Design review of the part built by this model. Coordinates are the model's own, in mm. A direction names the side the tool comes from. Round coordinates to 2 decimals unless told otherwise and drop trailing zeros. Loops run counter-clockwise (first coordinate to the right, second up) from the corner with the lowest first, then second, coordinate; pieces in that order, holes last. Notation, with made-up numbers: (33.5, 5.25) -> (40.5, 5.25) arc R7 ccw to (40.5, 12.25) -> close; hole circle Ø10 at (36, 2.5). An arc over 180 degrees is marked (long way). Use a Markdown table: item, result. Add a question column.
from build123d import *

# Parameters (mm, degrees)
SKETCH1_W            = 6.185857864
SKETCH1_H            = 7.5
BOSS_EXTRUDE1_DEPTH  = 4
FILLET1_R            = 2
M3_CLEARANCE_HOLE1_D = 3.2
SKETCH4_W            = 2
SKETCH4_H            = 0.481048
SKETCH4_H_2          = 1
CUT_EXTRUDE1_DEPTH   = 10
FILLET2_R            = 10
FILLET3_R            = 1
FILLET4_R            = 1


with BuildPart() as part:
    # Sketch1 → Boss-Extrude1 (new body)
    with BuildSketch(Plane.XY):
        Polygon((-4.235857864, -11.50026715), (-4.235857864, 0.5), (-19.56054874, 0.5), (-19.56054874, 9.2), (16.83945126, 9.2), (16.83945126, 0.5), (13.95, 0.5), (13.95, -7), (27.186678327, -7), (28.517391444, -8.547881241), (28.517391444, -11.5), align=None)
        with Locations((4.857071068, -3.25)):
            Rectangle(SKETCH1_W, SKETCH1_H, mode=Mode.SUBTRACT)
    extrude(amount=BOSS_EXTRUDE1_DEPTH)

    # Fillet1
    fillet1_edges = [part.edges().sort_by_distance(p)[0] for p in [
        (1.764142136, -7, 2),
        (7.95, -7, 2),
        (-4.235857864, -11.50026715, 2),
        (13.95, -7, 2),
        (28.517391444, -11.5, 2),
    ]]
    fillet(fillet1_edges, radius=FILLET1_R)

    # M3 Clearance Hole1 (through all)
    with Locations(Plane.XY.offset(4)):
        with Locations((10.95, -2.5), (-1.235857864, -2.5), (11.502527164, 5.109476), (-15.36054874, 5.109476)):
            Hole(M3_CLEARANCE_HOLE1_D / 2)

    # Sketch4 → Cut-Extrude1 (cut)
    with BuildSketch(Plane.XY.offset(4)):
        with Locations((8.502527164, 8.959476)):
            Rectangle(SKETCH4_W, SKETCH4_H)
        with Locations((-12.36054874, 8.959476)):
            Rectangle(SKETCH4_W, SKETCH4_H)
        with Locations((-12.36054874, 1)):
            Rectangle(SKETCH4_W, SKETCH4_H_2)
        Polygon((7.502527164, 0.5), (7.502527164, 1.5), (9.502527164, 1.5), (9.502527164, 0.5), (9.502527164, 0), (7.502527164, 0), align=None)
    extrude(amount=-CUT_EXTRUDE1_DEPTH, mode=Mode.SUBTRACT)

    # Fillet2
    # the kernel refuses this fillet: 10 mm, written as the material it takes off along each edge
    with BuildSketch(Plane(origin=(7.502527164, 0.5, -10.897247359), x_dir=(-1, 0, 0), z_dir=(0, 0, 1))) as fillet2_piece_1:
        with BuildLine():
            CenterArc((4.358898944, -10), FILLET2_R, 90, 25.841932763)
            Line((0, -1), (0, 0))
            Line((0, 0), (4.358898944, 0))
        make_face()
    extrude(amount=25.794494718, mode=Mode.SUBTRACT)
    with BuildSketch(Plane(origin=(7.95, 0, 16.650074726), x_dir=(1.0, -2.8096218791575343e-12, 0), z_dir=(0, 0, -1))) as fillet2_piece_2:
        with BuildLine():
            CenterArc((9.994593415, 5.36017886), FILLET2_R, 181.719985699, 30.692982598)
            Line((-0.000901098, 5.06002981), (-1.000450549, 5.030014905))
            ThreePointArc((-1.000450549, 5.030014905), (-1, 5), (-1, 0))
            Line((-1, 0), (0, -1))
            ThreePointArc((0, -1), (0.776263582, -1), (0.708320539, -0.536017886))
            Line((0.708320539, -0.536017886), (1.552527164, 0))
        make_face()
    extrude(amount=29.300149451, mode=Mode.SUBTRACT)

    # Fillet3
    # the kernel refuses this fillet: 1 mm, written as the material it adds along each edge
    with BuildSketch(Plane(origin=(9.502527164, 0, 4), x_dir=(0, 1, 0), z_dir=(0, 0, -1))) as fillet3_piece_1:
        with BuildLine():
            CenterArc((0.283169872, -1), FILLET3_R, 90, 30.865981789)
            ThreePointArc((-0.229861831, -0.141630341), (-0.114452906, -0.071590966), (0, 0))
            Line((0, 0), (0.283169872, 0))
        make_face()
    extrude(amount=4)
    with BuildSketch(Plane(origin=(9.502527164, 1.5, 4), x_dir=(-1, 0, 0), z_dir=(0, 0, -1))) as fillet3_piece_2:
        with BuildLine():
            CenterArc((FILLET3_R, -FILLET3_R), FILLET3_R, 90, 90)
            Line((0, -FILLET3_R), (0, 0))
            Line((0, 0), (FILLET3_R, 0))
        make_face()
    extrude(amount=4)
    with BuildSketch(Plane(origin=(7.502527164, 1.5, 4), x_dir=(-0.9045968857212806, -0.42626807802527333, 0), z_dir=(0, 0, -1))) as fillet3_piece_3:
        with BuildLine():
            CenterArc((0.223930785, -0.999943145), FILLET3_R, 90.610977717, 24.619977329)
            Line((-0.202337293, -0.095346259), (0, 0))
            ThreePointArc((0, 0), (0.106633707, -0.000568554), (0.213267415, 0))
        make_face()
    extrude(amount=4)
    with BuildSketch(Plane(origin=(-13.36054874, 8.718952, 4), x_dir=(0, 1, 0), z_dir=(0, 0, -1))) as fillet3_piece_4:
        with BuildLine():
            CenterArc((1, 0.854803382), FILLET3_R, 180, 58.738020049)
            Line((0, 0.854803382), (0, 0))
            Line((0, 0), (0.481048, 0))
        make_face()
    extrude(amount=4)
    with BuildSketch(Plane(origin=(-11.36054874, 8.718952, 4), x_dir=(-1, 0, 0), z_dir=(0, 0, -1))) as fillet3_piece_5:
        with BuildLine():
            CenterArc((0.854803382, 1), FILLET3_R, 211.261979951, 58.738020049)
            Line((0, 0.481048), (0, 0))
            Line((0, 0), (0.854803382, 0))
        make_face()
    extrude(amount=4)
    with BuildSketch(Plane(origin=(9.502527164, 8.718952, 4), x_dir=(0, 1, 0), z_dir=(0, 0, -1))) as fillet3_piece_6:
        with BuildLine():
            CenterArc((1, -0.854803382), FILLET3_R, 121.261979951, 58.738020049)
            Line((0, -0.854803382), (0, 0))
            Line((0, 0), (0.481048, 0))
        make_face()
    extrude(amount=4)
    with BuildSketch(Plane(origin=(7.502527164, 8.718952, 4), x_dir=(1, 0, 0), z_dir=(0, 0, -1))) as fillet3_piece_7:
        with BuildLine():
            CenterArc((0.854803382, -1), FILLET3_R, 90, 58.738020049)
            Line((0, -0.481048), (0, 0))
            Line((0, 0), (0.854803382, 0))
        make_face()
    extrude(amount=4)
    with BuildSketch(Plane(origin=(-13.36054874, 1.5, 4), x_dir=(1, 0, 0), z_dir=(0, 0, -1)), Plane(origin=(-11.36054874, 1.5, 4), x_dir=(0, -1, 0), z_dir=(0, 0, -1))) as fillet3_piece_8:
        with BuildLine():
            CenterArc((FILLET3_R, FILLET3_R), FILLET3_R, 180, 90)
            Line((0, FILLET3_R), (0, 0))
            Line((0, 0), (FILLET3_R, 0))
        make_face()
    extrude(amount=4)
    # the kernel refuses this fillet: 1 mm, written as the material it takes off along each edge
    with BuildSketch(Plane(origin=(28.517391444, -8.547881241, -0.926902713), x_dir=(0, -1, 0), z_dir=(0, 0, 1))) as fillet3_2_piece_1:
        with BuildLine():
            CenterArc((FILLET3_R * 0.370761085346, -FILLET3_R), FILLET3_R, 90, 40.685640486)
            Line((-FILLET3_R * 0.28114729377, -FILLET3_R * 0.241702258187), (0, 0))
            Line((0, 0), (FILLET3_R * 0.370761085346, 0))
        make_face()
    extrude(amount=5.853805427, mode=Mode.SUBTRACT)
    with BuildSketch(Plane(origin=(27.186678327, -7, -1.147608656), x_dir=(0.6519083791154829, -0.7582977418132165, 0), z_dir=(0, 0, 1))) as fillet3_2_piece_2:
        with BuildLine():
            CenterArc((FILLET3_R * 0.459043462337, -FILLET3_R), FILLET3_R, 90, 49.314359514)
            Line((-FILLET3_R * 0.299254279476, -FILLET3_R * 0.348091620885), (0, 0))
            Line((0, 0), (FILLET3_R * 0.459043462337, 0))
        make_face()
    extrude(amount=6.295217312, mode=Mode.SUBTRACT)
    with BuildSketch(Plane(origin=(-19.56054874, 0.5, -2.5), x_dir=(0, 1, 0), z_dir=(0, 0, 1)), Plane(origin=(-19.56054874, 9.2, -2.5), x_dir=(1, 0, 0), z_dir=(0, 0, 1)), Plane(origin=(16.83945126, 9.2, -2.5), x_dir=(0, -1, 0), z_dir=(0, 0, 1)), Plane(origin=(16.83945126, 0.5, -2.5), x_dir=(-1, 0, 0), z_dir=(0, 0, 1))) as fillet3_2_piece_3:
        with BuildLine():
            CenterArc((FILLET3_R, -FILLET3_R), FILLET3_R, 90, 90)
            Line((0, -FILLET3_R), (0, 0))
            Line((0, 0), (FILLET3_R, 0))
        make_face()
    extrude(amount=9, mode=Mode.SUBTRACT)

    # Fillet4
    fillet4_edges = [part.edges().sort_by_distance(p)[0] for p in [
        (9.502527164, 9.2, 2),
        (7.502527164, 9.2, 2),
        (-11.36054874, 9.2, 2),
        (-13.36054874, 9.2, 2),
        (-13.36054874, 0.5, 2),
        (-11.36054874, 0.5, 2),
    ]]
    fillet(fillet4_edges, radius=FILLET4_R)


solid = part.part
1. Insertion check: P1, Ø1.9, axis at x = 11.5, y = 5.11, coming from the +Z side; P2, Ø1.2, axis at y = -4, z = 2.5, coming from the -X side; P3, Ø1.2, axis at y = -3, z = 1.5, coming from the +X side; P4, Ø2, axis at x = 23.5, z = 1.5, coming from the +Y side. Each pin has a flat end and moves straight along its axis. Give the tip position at first contact, or say it passes through.
2. Consider section A-A on y = -2.5. State the section outline as (x, z) points, plus the area to 3 significant figures.
3. To check wall thickness, follow probe 1 along X at (y, z) = (6.25, 2.8); probe 2 along X at (y, z) = (1.25, 1.25); probe 3 along Y at (x, z) = (24, 3.45). State the ranges of each line that lie inside material, in increasing order. Write a range as from..to.
4. For faces 1 (the face through (15, 0.5, 2)), 2 (the face through (5, 1, 0)), 3 (the face through (-7, 0.5, 2)), 4 (the face through (16.839, 5, 2)), 5 (the face through (9.202, 1.215, 2.028)), list the 3-axis set-ups (+Z, -Z, +X, -X, +Y, -Y) from which the entire face can be reached by the end or side of a thin tool; tool diameter is ignored.
5. Consider section C-C on x = -7.5. State the section outline as (y, z) points, plus the area to 3 significant figures.
6. Consider section B-B on x = 10.95. State the section outline as (y, z) points, plus the area to 3 significant figures.
7. Mouldability with a two-part tool opening along Y and no side actions: class faces 6 (the face through (-4.236, -5, 2)), 7 (the face through (-16, 9.2, 2)), 8 (the face through (2, 0.5, 2)) as +Y half, -Y half, draft (parallel to the pull), parting line (faces both ways), or undercut.
8. Consider section D-D on z = 1.2. Give the number of separate pieces and of enclosed holes in the cut face, plus the area to 3 significant figures.
Verdict:
| question | item | result |
|---|---|---|
| 1 | P1 | passes through |
| 1 | P2 | stops at x = -4.24 |
| 1 | P3 | stops at x = 13.95 |
| 1 | P4 | stops at y = -7 |
| 2 | outline | (-4.24, 0) -> (-2.84, 0) -> (-2.84, 4) -> (-4.24, 4) -> close; (0.36, 0) -> (1.76, 0) -> (1.76, 4) -> (0.36, 4) -> close; (8.36, 0) -> (9.35, 0) -> (9.35, 4) -> (8.36, 4) -> close; (12.55, 0) -> (13.95, 0) -> (13.95, 4) -> (12.55, 4) -> close |
| 2 | area | 20.8 mm² |
| 3 | probe 1 | x = -19.56..-16.48, -14.24..10.38, 12.62..16.84 |
| 3 | probe 2 | x = -19.53..-13.02, -11.7..6.94, 9.16..16.81 |
| 3 | probe 3 | y = -11.5..-7 |
| 4 | face 1 | +Z, -Z, +X |
| 4 | face 2 | -Z, +X, -X, +Y, -Y |
| 4 | face 3 | +Z, -Z, -X, -Y |
| 4 | face 4 | +Z, -Z, +X, +Y |
| 4 | face 5 | +Z, -Z |
| 5 | outline | (0.5, 0) -> (9.2, 0) -> (9.2, 4) -> (0.5, 4) -> close |
| 5 | area | 34.8 mm² |
| 6 | outline | (-11.5, 0) -> (-4.1, 0) -> (-4.1, 4) -> (-11.5, 4) -> close; (-0.9, 0) -> (3.61, 0) -> (3.61, 4) -> (-0.9, 4) -> close; (6.61, 0) -> (9.2, 0) -> (9.2, 4) -> (6.61, 4) -> close |
| 6 | area | 58.0 mm² |
| 7 | face 6 | draft |
| 7 | face 7 | +Y half |
| 7 | face 8 | undercut |
| 8 | separate pieces | 1 |
| 8 | enclosed holes | 5 |
| 8 | area | 511 mm² |
